Could you check a few things on this model? Use its own coordinates, in mm. A direction names the side the tool comes from. Coordinates: 2 decimals unless noted, no trailing zeros. Loops run counter-clockwise (first coordinate to the right, second up) from the corner with the lowest first, then second, coordinate; pieces in that order, holes last. Notation, with made-up numbers: (-23.5, 34.25) -> (5.5, 34.25) arc R34 ccw to (5.5, 68.25) -> close; hole circle Ø10 at (-40, -22). An arc over 180 degrees is marked (long way). One line per question, with ' | ' between items.
from build123d import *

# Parameters (mm, degrees)
F0_R     = 8.5
F0_W     = 6.55
F0_H     = 6.55
F1_DEPTH = 33
F3_DEPTH = 25
F4_R     = 7.25
F5_DEPTH = 23


with BuildPart() as f1:
    # F0 (on Front) → F1 (new body)
    with BuildSketch(Plane.XZ):
        Circle(F0_R)
        Rectangle(F0_W, F0_H, mode=Mode.SUBTRACT)
    extrude(amount=F1_DEPTH)

    # F2 (on face) → F3 (cut)
    with BuildSketch(Plane.XZ.offset(33)):
        Polygon((-3.275, -3.243106), (-3.275, 2.389649), (-4.451013, 1.233619), (-3.293852, -3.237881), align=None)
        Polygon((1.157162, -4.4715), (2.374344, -3.275), (-3.159923, -3.275), align=None)
        Polygon((4.451013, -1.233619), (3.293852, 3.237881), (3.275, 3.243106), (3.275, -2.389649), align=None)
        Polygon((-2.374344, 3.275), (3.159923, 3.275), (-1.157162, 4.4715), align=None)
    extrude(amount=-F3_DEPTH, mode=Mode.SUBTRACT)

    # F4 (on face) → F5 (cut)
    with BuildSketch(Plane.XZ.offset(33)):
        Circle(F4_R)
        Polygon((-1.157162, 4.4715), (3.159923, 3.275), (3.275, 3.275), (3.275, 3.243106), (3.293852, 3.237881), (4.451013, -1.233619), (3.275, -2.389649), (3.275, -3.275), (2.374344, -3.275), (1.157162, -4.4715), (-3.159923, -3.275), (-3.275, -3.275), (-3.275, -3.243106), (-3.293852, -3.237881), (-4.451013, 1.233619), (-3.275, 2.389649), (-3.275, 3.275), (-2.374344, 3.275), align=None, mode=Mode.SUBTRACT)
    extrude(amount=-F5_DEPTH, mode=Mode.SUBTRACT)


solid = f1.part
1) If we section it at B-B on y = -6: Please give me the cut outline in (x, z) (3 decimals), and give its area (3 significant figures).
Data:
outline: circle Ø17 at (0, 0); hole (-3.275, -3.275) -> (3.275, -3.275) -> (3.275, 3.275) -> (-3.275, 3.275) -> close | area: 184 mm²
2) We'd pull the mould along Z, two halves only. Please class faces 3 (the face through (4.57, -16.269, 7.167)), 4 (the face through (-1.032, -9.014, -3.865)), 5 (the face through (7, -33, 3)): pulls with the +Z half, pulls with the -Z half, needs draft (parallel to the pull), parting line crosses it, or undercut.
Data:
face 3: parting line crosses it | face 4: undercut | face 5: needs draft
3) I need wall thicknesses on line 1 along Z through (x, y) = (0, -15.5); line 2 along X through (y, z) = (-5, 0.25) (3 decimals); line 3 along Y through (x, z) = (3.75, -1.5). Which ranges of each line are inside material? Lowest first, please. Write a range as from..to.
Data:
line 1: -8.5..-7.25, 7.25..8.5 | line 2: -8.496..-3.275, 3.275..8.496 | line 3: -8..0
4) I'm going to push flat-ended pins straight in: pin 1 Ø4.5 at (x, z) = (-3.5, -2.5) entering from -Y; pin 2 Ø4 at (x, y) = (2.5, -6.5) entering from -Z; pin 3 Ø8 at (x, y) = (5, -19) entering from +Z. Where does each tip first touch, or does it pass through?
Data:
pin 1: y = -10 | pin 2: z = -8.49 | pin 3: z = 8.44
5) If we section it at D-D on x = 5: Please give me the cut outline in (y, z), and give its area (3 significant figures).
Data:
outline: (-33, -6.87) -> (0, -6.87) -> (0, 6.87) -> (-33, 6.87) -> (-33, 5.25) -> (-10, 5.25) -> (-10, -5.25) -> (-33, -5.25) -> close | area: 212 mm²
6) On a 3-axis mill with a long thin cutter (end or side, diameter ignored), from which of +Z, -Z, +X, -X, +Y, -Y can I reach the whole of each face in a straight line? I mean faces 1 (the face through (3.855, -9.014, -1.82)), 2 (the face through (-3.275, -4, 0)). Say none if no direction works.
Data:
face 1: -Y | face 2: +Y, -Y
7) If we section it at C-C on x = 0: Please give me the cut outline in (y, z) (3 decimals), and give its area (3 significant figures).
Data:
outline: (-33, -8.5) -> (0, -8.5) -> (0, -3.275) -> (-8, -3.275) -> (-8, -4.151) -> (-10, -4.151) -> (-10, -7.25) -> (-33, -7.25) -> close; (-33, 7.25) -> (-10, 7.25) -> (-10, 4.151) -> (-8, 4.151) -> (-8, 3.275) -> (0, 3.275) -> (0, 8.5) -> (-33, 8.5) -> close | area: 158 mm²
8) If we section it at A-A on z = 0: Please give me the cut outline in (x, y) (3 decimals), and give its area (3 significant figures).
Data:
outline: (-8.5, -33) -> (-7.25, -33) -> (-7.25, -10) -> (-4.132, -10) -> (-4.132, -8) -> (-3.275, -8) -> (-3.275, 0) -> (-8.5, 0) -> close; (3.275, -8) -> (4.132, -8) -> (4.132, -10) -> (7.25, -10) -> (7.25, -33) -> (8.5, -33) -> (8.5, 0) -> (3.275, 0) -> close | area: 159 mm²
